Could you check a few things on this model? Use its own coordinates, in mm. A direction names the side the tool comes from. Coordinates: 2 decimals unless noted, no trailing zeros. Order: outer loops, then holes, each group sorted by start corner. A loop starts at its lowest first (then second) coordinate and runs counter-clockwise, first axis right, second up. Notation, with made-up numbers: (82.25, 68) -> (91.25, 68) arc R5 cw to (91.25, 75) -> close; hole circle Ø5 at (42, 60). An arc over 180 degrees is marked (long way). Use a Markdown table: item, result. Add a question column.
1) If we section it at B-B (x = 39): Write out the boundary of the cut face in (y, z).
2) If we section it at C-C (y = -0.75): Write out the boundary of the cut face in (x, z), plus the area to 3 significant figures.
3) If we section it at D-D (z = 8): Write out the boundary of the cut face in (x, y).
4) Which directions (+Z, -Z, +X, -X, +Y, -Y) give clear straight access to the entire face, cutting with the end or side of a thin tool? Please do faces 4 (the flat face through (37, -1, -5)), 5 (the flat face through (5.237, -1, -11)), 6 (the flat face through (17.4, -1.5, 15.8)), 7 (the flat face through (37, -3, 9)), 8 (the flat face through (3, 12, 0)).
5) Will these pins go through, and if not, where does the flat tip stop? pin 1 Ø1.6 at (x, y) = (2.5, 10) entering from +Z; pin 2 Ø1 at (y, z) = (9.5, 5) entering from +X; pin 3 Ø0.6 at (x, y) = (5, -1) entering from -Z.
6) If we section it at A-A (z = 0): Write out the boundary of the cut face in (x, y), plus the area to 3 significant figures.
7) If I drill on L1, parallel to Z at x = 49, y = -2; L2, parallel to X at y = 1, z = 7.5; L3, parallel to Y at x = 54, z = -18, over which ranges is the centre line in solid material (lowest first)? Write a range as [from, to].
8) Thinking about a two-plate mould opening in X: for faces 1 (the flat face through (70, -1, 0)), 2 (the flat face through (1, 10, 10)), 3 (the cylindrical face through (20, -1, 0)), which applies, +X half, -X half, draft (parallel to the pull), parting line (faces both ways), or undercut?
```python
from build123d import *

# Parameters (mm, degrees)
BASE_FLANGE1_DEPTH            = 3
EDGE_FLANGE1_STRIP_W          = 13.4732
EDGE_FLANGE1_STRIP_H          = 3
EDGE_FLANGE1_STRIP_CUT_DEPTH  = 20
EDGE_FLANGE1_RELIEF_W         = 14.9732
EDGE_FLANGE1_RELIEF_H         = 1.5
EDGE_FLANGE1_RELIEF_CUT_DEPTH = 3
EDGE_FLANGE1_DEPTH            = 20
CUT_EXTRUDE1_DEPTH            = 10


# Sheet-metal steps are written as plain solids
with BuildPart() as part:
    # Sketch1 → Base-Flange1 (new body)
    with BuildSketch(Plane(origin=(0, 0, 0), x_dir=(1, 0, 0), z_dir=(0, 1, 0))):
        Polygon((0, 0), (0, 10), (30, 20), (70, 20), (70, 0), (70, -20), (30, -20), (0, -10), align=None)
    extrude(amount=-BASE_FLANGE1_DEPTH)

    # Edge-Flange1 strip (across the edge) → Edge-Flange1 strip cut (cut)
    with BuildSketch(Plane.XY.offset(-10)):
        with Locations((-3, -1.5)):
            Rectangle(EDGE_FLANGE1_STRIP_W, EDGE_FLANGE1_STRIP_H)
    extrude(amount=EDGE_FLANGE1_STRIP_CUT_DEPTH, mode=Mode.SUBTRACT)

    # Edge-Flange1 relief (on the sheet) → Edge-Flange1 relief cut (cut)
    with BuildSketch(Plane(origin=(3.7366, 0, -10), x_dir=(1, 0, 0), z_dir=(0, 1, 0))):
        with Locations((-5.9866, 0.75)):
            Rectangle(EDGE_FLANGE1_RELIEF_W, EDGE_FLANGE1_RELIEF_H)
        with Locations((-5.9866, -20.75)):
            Rectangle(EDGE_FLANGE1_RELIEF_W, EDGE_FLANGE1_RELIEF_H)
    extrude(amount=-EDGE_FLANGE1_RELIEF_CUT_DEPTH, mode=Mode.SUBTRACT)

    # Edge-Flange1 section (across the edge) → Edge-Flange1 (add)
    with BuildSketch(Plane.XY.offset(-10)):
        with BuildLine():
            Line((0, 0.7366), (0, 22))
            Line((0, 22), (3, 22))
            Line((3, 22), (3, 0.7366))
            ThreePointArc((3, 0.7366), (3.215745145, 0.215745145), (3.7366, 0))
            Line((3.7366, 0), (3.7366, -3))
            ThreePointArc((3.7366, -3), (1.094424801, -1.905575199), (0, 0.7366))
        make_face()
    extrude(amount=EDGE_FLANGE1_DEPTH)

    # Sketch9 → Cut-Extrude1 (cut)
    with BuildSketch(Plane(origin=(0, 0, 0), x_dir=(1, 0, 0), z_dir=(0, 1, 0))):
        with BuildLine():
            Line((50, -5), (25, -5))
            ThreePointArc((25, -5), (20, 0), (25, 5))
            Line((25, 5), (50, 5))
            ThreePointArc((50, 5), (55, 0), (50, -5))
        make_face()
    extrude(amount=-CUT_EXTRUDE1_DEPTH, mode=Mode.SUBTRACT)


solid = part.part
```
Answer sheet:
| question | item | result |
|---|---|---|
| 1 | outline | (-3, -20) -> (0, -20) -> (0, -5) -> (-3, -5) -> close; (-3, 5) -> (0, 5) -> (0, 20) -> (-3, 20) -> close |
| 2 | outline | (0.31, -10) -> (5.24, -10) -> (5.24, -11.5) -> (4.5, -11.5) -> (30, -20) -> (70, -20) -> (70, 20) -> (30, 20) -> (4.5, 11.5) -> (5.24, 11.5) -> (5.24, 10) -> (0.31, 10) -> close; hole (25, -5) -> (50, -5) arc R5 ccw to (50, 5) -> (25, 5) arc R5 ccw to start |
| 2 | area | 2,160 mm2 |
| 3 | outline | (0, 0.74) arc R3.74 ccw to (3.74, -3) -> (70, -3) -> (70, 0) -> (3.74, 0) arc R0.74 cw to (3, 0.74) -> (3, 22) -> (0, 22) -> close |
| 4 | face 4 | +Y, -Y |
| 4 | face 5 | -X, +Y, -Y |
| 4 | face 6 | +Z, -X, +Y, -Y |
| 4 | face 7 | +Z, -Z, +X, -X, -Y |
| 4 | face 8 | +Z, -Z, +X, +Y |
| 5 | pin 1 | z = 10 |
| 5 | pin 2 | x = 3 |
| 5 | pin 3 | z = -11.77 |
| 6 | outline | (0, 0.74) arc R3.74 ccw to (3.74, -3) -> (20, -3) -> (20, 0) -> (3.74, 0) arc R0.74 cw to (3, 0.74) -> (3, 22) -> (0, 22) -> close; (55, -3) -> (70, -3) -> (70, 0) -> (55, 0) -> close |
| 6 | area | 168 mm2 |
| 7 | L1 | [-20, -5], [5, 20] |
| 7 | L2 | [0, 3] |
| 7 | L3 | [-3, 0] |
| 8 | face 1 | +X half |
| 8 | face 2 | draft |
| 8 | face 3 | undercut |
